Could you check a few things on this model? Use its own coordinates, in mm. A direction names the side the tool comes from. Coordinates: 2 decimals unless noted, no trailing zeros. Order: outer loops, then holes, each group sorted by start corner. A loop starts at its lowest first (then second) coordinate and runs counter-clockwise, first axis right, second up. Notation, with made-up numbers: (62.25, 39.5) -> (69.25, 39.5) arc R28 cw to (69.25, 71.5) -> close; hole circle Ø1 at (18.5, -9.5). An arc over 180 degrees is marked (long way). Use a Markdown table: item, result. Add a question column.
1) If we section it at B-B (y = 118.5): Write out the boundary of the cut face in (x, z), plus the area to 3 significant figures.
2) If we section it at D-D (y = 148.5): Write out the boundary of the cut face in (x, z), plus the area to 3 significant figures.
3) If I drill on L1, parallel to Y at x = 94.5, z = -1; L2, parallel to X at y = 159, z = -0.25; L3, parallel to Y at x = 150, z = -1.75, over which ranges is the centre line in solid material (lowest first)? Write a range as [from, to].
4) Which directions (+Z, -Z, +X, -X, +Y, -Y) give clear straight access to the entire face, cutting with the end or side of a thin tool? Please do faces 1 (the flat face through (209.14, 147, -3)), 2 (the flat face through (133, 119.722, -3)), 3 (the flat face through (118.653, 158, -3)).
5) If we section it at A-A (x = 114): Write out the boundary of the cut face in (y, z), plus the area to 3 significant figures.
6) Thinking about a two-plate mould opening in Y: for faces 4 (the flat face through (142, 113.372, -3)), 5 (the flat face through (92, 151.472, -3)), 6 (the flat face through (161, 160.997, -3)), which applies, +Y half, -Y half, draft (parallel to the pull), parting line (faces both ways), or undercut?
7) Will these pins go through, and if not, where does the flat tip stop? pin 1 Ø1.5 at (y, z) = (124, -1.5) entering from -X; pin 2 Ø3 at (x, z) = (113, -3) entering from -Y; pin 3 Ø3 at (x, z) = (133, -4) entering from +Y.
8) If we section it at C-C (y = 143.5): Write out the boundary of the cut face in (x, z), plus the area to 3 significant figures.
```python
from build123d import *

# Parameters (mm, degrees)
SKETCH1_W           = 127
SKETCH1_H           = 47.625
BOSS_EXTRUDE1_DEPTH = 6.35
SKETCH2_W           = 9.525
SKETCH2_H           = 12.7
CUT_EXTRUDE1_DEPTH  = 270.065952098
LPATTERN1_COUNT     = 3
LPATTERN1_PITCH     = 19.05
LPATTERN1_COL_COUNT = 3
LPATTERN1_COL_PITCH = 19.05
CUT_EXTRUDE3_DEPTH  = 270.065952098
CAVITY1_START       = 122.897475598
CAVITY1_OUTLINE_W   = 6.35
CAVITY1_OUTLINE_H   = 6.35
CAVITY1_DEPTH       = 9.525
CAVITY1_START_2     = 141.947475598
CAVITY1_2_OUTLINE_W = 6.35
CAVITY1_2_OUTLINE_H = 6.35
CAVITY1_2_DEPTH     = 9.525


# Read off the part's stored shape, not the designer's step: Cavity1
with BuildPart() as part:
    # Sketch1 → Boss-Extrude1 (new body)
    with BuildSketch(Plane.XY):
        with Locations((151.990085455, 137.184975598)):
            Rectangle(SKETCH1_W, SKETCH1_H)
    extrude(amount=-BOSS_EXTRUDE1_DEPTH)

    # Sketch2 → Cut-Extrude1 (cut, through all)
    with BuildSketch(Plane(origin=(0, 0, -6.35), x_dir=(-1, 0, 0), z_dir=(0, 0, -1))):
        with Locations((-151.990085455, 160.997475598)):
            Rectangle(SKETCH2_W, SKETCH2_H)
        with Locations((-151.990085455, 113.372475598)):
            Rectangle(SKETCH2_W, SKETCH2_H)
    cut_extrude1 = extrude(amount=-CUT_EXTRUDE1_DEPTH, mode=Mode.SUBTRACT)

    # LPattern1: Cut-Extrude1 ×3
    with Locations(*[(-i * LPATTERN1_PITCH, 0, 0) for i in range(1, LPATTERN1_COUNT)]):
        add(cut_extrude1, mode=Mode.SUBTRACT)

    # LPattern1 col: Cut-Extrude1 ×3
    with Locations(*[(i * LPATTERN1_COL_PITCH, 0, 0) for i in range(1, LPATTERN1_COL_COUNT)]):
        add(cut_extrude1, mode=Mode.SUBTRACT)

    # Sketch3 → Cut-Extrude3 (cut, through all)
    with BuildSketch(Plane(origin=(0, 0, -6.35), x_dir=(-1, 0, 0), z_dir=(0, 0, -1))):
        with BuildLine():
            Line((-193.265085455, 145.122475598), (-110.715085455, 145.122475598))
            ThreePointArc((-110.715085455, 145.122475598), (-102.777585455, 137.184975598), (-110.715085455, 129.247475598))
            Line((-110.715085455, 129.247475598), (-193.265085455, 129.247475598))
            ThreePointArc((-193.265085455, 129.247475598), (-201.202585455, 137.184975598), (-193.265085455, 145.122475598))
        make_face()
    extrude(amount=-CUT_EXTRUDE3_DEPTH, mode=Mode.SUBTRACT)

    # Cavity1 outline → Cavity1 (cut)
    with BuildSketch(Plane(origin=(0, 0, 0), x_dir=(1, 0, 0), z_dir=(0, 1, 0)).offset(CAVITY1_START)):
        with Locations((91.665085455, 3.175)):
            Rectangle(CAVITY1_OUTLINE_W, CAVITY1_OUTLINE_H)
        with Locations((212.315085455, 3.175)):
            Rectangle(CAVITY1_OUTLINE_W, CAVITY1_OUTLINE_H)
    extrude(amount=CAVITY1_DEPTH, mode=Mode.SUBTRACT)

    # Cavity1 2 outline → Cavity1 2 (cut)
    with BuildSketch(Plane(origin=(0, 0, 0), x_dir=(1, 0, 0), z_dir=(0, 1, 0)).offset(CAVITY1_START_2)):
        with Locations((91.665085455, 3.175)):
            Rectangle(CAVITY1_2_OUTLINE_W, CAVITY1_2_OUTLINE_H)
        with Locations((212.315085455, 3.175)):
            Rectangle(CAVITY1_2_OUTLINE_W, CAVITY1_2_OUTLINE_H)
    extrude(amount=CAVITY1_2_DEPTH, mode=Mode.SUBTRACT)


solid = part.part
```
Answer sheet:
| question | item | result |
|---|---|---|
| 1 | outline | (88.49, -6.35) -> (109.13, -6.35) -> (109.13, 0) -> (88.49, 0) -> close; (118.65, -6.35) -> (128.18, -6.35) -> (128.18, 0) -> (118.65, 0) -> close; (137.7, -6.35) -> (147.23, -6.35) -> (147.23, 0) -> (137.7, 0) -> close; (156.75, -6.35) -> (166.28, -6.35) -> (166.28, 0) -> (156.75, 0) -> close; (175.8, -6.35) -> (185.33, -6.35) -> (185.33, 0) -> (175.8, 0) -> close; (194.85, -6.35) -> (215.49, -6.35) -> (215.49, 0) -> (194.85, 0) -> close |
| 1 | area | 504 mm2 |
| 2 | outline | (94.84, -6.35) -> (209.14, -6.35) -> (209.14, 0) -> (94.84, 0) -> close |
| 2 | area | 726 mm2 |
| 3 | L1 | [113.37, 122.9], [132.42, 141.95], [151.47, 161] |
| 3 | L2 | [88.49, 109.13], [118.65, 128.18], [137.7, 147.23], [156.75, 166.28], [175.8, 185.33], [194.85, 215.49] |
| 3 | L3 | [119.72, 129.25], [145.12, 154.65] |
| 4 | face 1 | +Z, -Z, +X |
| 4 | face 2 | +Z, -Z, -Y |
| 4 | face 3 | +Z, -Z, +Y |
| 5 | outline | (119.72, -6.35) -> (129.25, -6.35) -> (129.25, 0) -> (119.72, 0) -> close; (145.12, -6.35) -> (154.65, -6.35) -> (154.65, 0) -> (145.12, 0) -> close |
| 5 | area | 121 mm2 |
| 6 | face 4 | -Y half |
| 6 | face 5 | undercut |
| 6 | face 6 | +Y half |
| 7 | pin 1 | x = 94.84 |
| 7 | pin 2 | y = 119.72 |
| 7 | pin 3 | y = 154.65 |
| 8 | outline | (94.84, -6.35) -> (105.91, -6.35) -> (105.91, 0) -> (94.84, 0) -> close; (198.07, -6.35) -> (209.14, -6.35) -> (209.14, 0) -> (198.07, 0) -> close |
| 8 | area | 141 mm2 |
